Model file for the job. Use its own axes, mm. A direction names the side the tool comes from. Give positions to 0.01 mm unless a question says otherwise; leave off trailing zeros. Loops run counter-clockwise (first coordinate to the right, second up) from the corner with the lowest first, then second, coordinate; pieces in that order, holes last. Notation, with made-up numbers: (37.5, 10) -> (49.5, 10) arc R19 cw to (49.5, 32) -> close; hole circle Ø11 at (83.25, 80). An arc over 180 degrees is marked (long way). Use CSV: the item, a comma, the result in double quotes. Start each with the question number.
(1) Pull direction X, two halves, no side cores. Call faces 1 (the flat face through (3, -2, 11)), 2 (the cylindrical face through (4.626, 1.457, 9.226)), 3 (the cylindrical face through (0.74, 3.32, 5.58)): pulls with the +X half, pulls with the -X half, needs draft (parallel to the pull), parting line crosses it, or undercut.
(2) 3-axis set-ups, long thin cutter, end or side, ignore diameter. For faces 4 (the flat face through (2, -5, 7.5)), 5 (the cylindrical face through (-2.38, -10.74, 3.7)): which of +Z, -Z, +X, -X, +Y, -Y reach the whole face in a straight line?
(3) Drill centre lines: probe 1 along Z at (x, y) = (4.75, -7.5); probe 2 along Y at (x, z) = (0, 2.5); probe 3 along X at (y, z) = (-1.5, 10.75). Where is each one in solid material? Low to high.
(4) Cut at D-D on x = 4.5. Write the cut outline in (y, z), then the cut area to 3 significant figures.
(5) Cut at C-C on z = 3.5. Write the cut outline in (x, y).
(6) Flat gauge pins, fed straight in: pin 1 (5 mm diameter, centred on x = -5, z = 3.5, fed in from +Y); pin 2 (1.5 mm diameter, centred on y = -6, z = 6, fed in from +X); pin 3 (1.5 mm diameter, centred on x = -7.5, z = 6, fed in from -Y). Where does each tip first touch, or does it go through?
(7) Cut at A-A on y = 0. Write the cut outline in (x, z).
from build123d import *

# Parameters (mm, degrees)
F0_R     = 11
F0_R_2   = 4.85
F1_DEPTH = 7.5
F2_DEPTH = 11
F3_D     = 6.8


with BuildPart() as f1:
    # F0 (on Top) → F1 (new body)
    with BuildSketch(Plane.XY):
        Circle(F0_R)
        Circle(F0_R_2, mode=Mode.SUBTRACT)
        Circle(F0_R_2)
    extrude(amount=F1_DEPTH)

    # F0 (on Top) → F2 (join)
    with BuildSketch(Plane.XY):
        Circle(F0_R_2)
    extrude(amount=F2_DEPTH)

    # F3 (through all)
    with Locations(Plane(origin=(0, 0, 0), x_dir=(1, 0, 0), z_dir=(0, 0, -1))):
        with Locations((0, 0)):
            Hole(F3_D / 2)


solid = f1.part
Check result:
1,face 1,"needs draft"
1,face 2,"parting line crosses it"
1,face 3,"undercut"
2,face 4,"+Z"
2,face 5,"+Z, -Z"
3,probe 1,"0 to 7.5"
3,probe 2,"-11 to -3.4, 3.4 to 11"
3,probe 3,"-4.61 to -3.05, 3.05 to 4.61"
4,outline,"(-10.04, 0) -> (10.04, 0) -> (10.04, 7.5) -> (1.81, 7.5) -> (1.81, 11) -> (-1.81, 11) -> (-1.81, 7.5) -> (-10.04, 7.5) -> close"
4,area,"163 mm²"
5,outline,"circle Ø22 at (0, 0); hole circle Ø6.8 at (0, 0)"
6,pin 1,"y = 10.71"
6,pin 2,"x = 9.67"
6,pin 3,"y = -8.69"
7,outline,"(-11, 0) -> (-3.4, 0) -> (-3.4, 11) -> (-4.85, 11) -> (-4.85, 7.5) -> (-11, 7.5) -> close; (3.4, 0) -> (11, 0) -> (11, 7.5) -> (4.85, 7.5) -> (4.85, 11) -> (3.4, 11) -> close"
